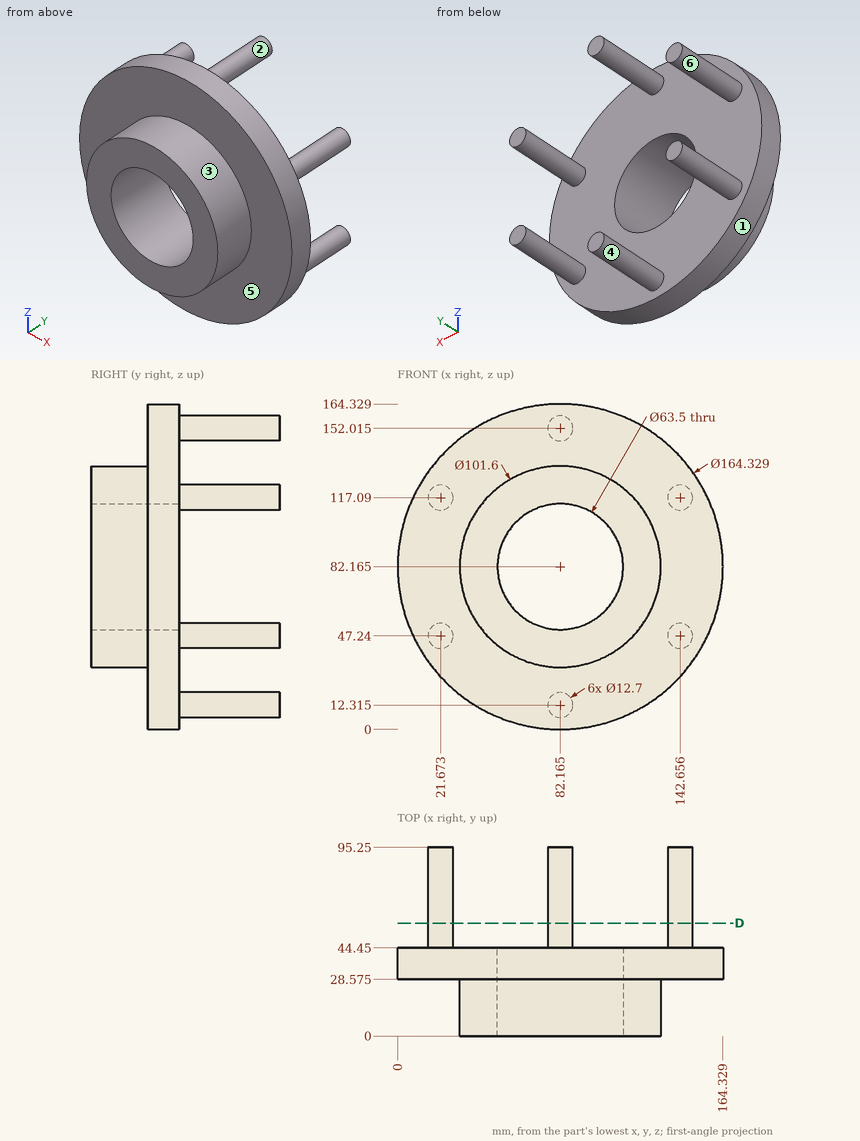
Drawing for the job (mm, zero at the part's lowest x, y, z). A direction names the side the tool comes from. Give positions to 0.01 mm unless a question says otherwise; leave off trailing zeros.
1) 3-axis set-ups, long thin cutter, end or side, ignore diameter. For the marked faces 1, 2 and 3: which of +Z, -Z, +X, -X, +Y, -Y reach the whole face in a straight line?
Values follow:
face 1: +Y, -Y
face 2: +Y
face 3: -Y
2) Two-plate mould, pull along X, no slides. Class the marked faces 4, 5 and 6: released by +X, released by -X, zero draft, split by the parting line, or undercut.
Values follow:
face 4: split by the parting line
face 5: zero draft
face 6: undercut
3) Band-saw the part on D-D on y = 57. State how many separate pieces and enclosed holes the cut face has, then the cut area to 3 significant figures.
Values follow:
separate pieces: 6
enclosed holes: 0
area: 760 mm2
4) Probe line 1 along Y through (x, z) = (119.5, 49); line 2 along Z through (x, y) = (53.5, 23.5) (1 decimal); line 3 along X through (y, z) = (34, 98.5). List the from-to ranges inside material, lowest first.
Values follow:
line 1: y = 0 to 44.45
line 2: z = 40.2 to 68.5, 95.8 to 124.1
line 3: x = 1.64 to 54.94, 109.39 to 162.69
5) Drop flat-ended pins along their axis: P1, Ø3, axis at x = 141, y = 64, coming from the -Z side; P2, Ø3, axis at x = 88, y = 74, coming from the -Z side (1 decimal); P3, Ø2, axis at x = 58.5, y = 29.5, coming from the +Z side; P4, Ø2, axis at x = 112.5, z = 61.5, coming from the -Y side. Give the stop position or say it passes through.
Values follow:
P1: stops at z = 40.89
P2: stops at z = 7.7
P3: stops at z = 161.14
P4: stops at y = 0
